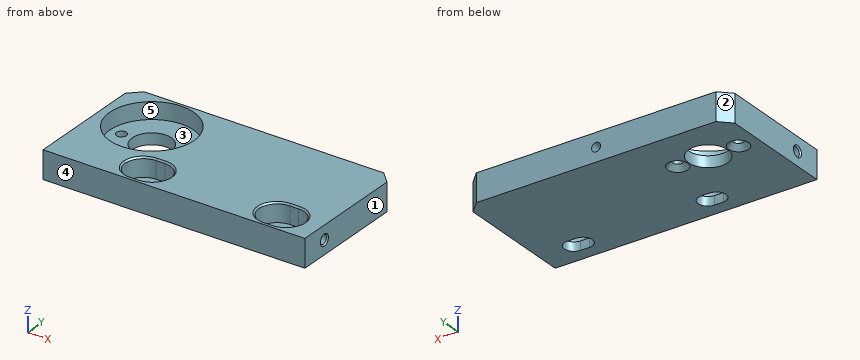
```python
from build123d import *

# Parameters (mm, degrees)
SKIZZE1_W                                            = 47
SKIZZE1_H                                            = 23
AUFSATZ_LINEAR_AUSTRAGEN1_DEPTH                      = 5
SKIZZE2_R                                            = 7.55
SCHNITT_LINEAR_AUSTRAGEN1_DEPTH                      = 3
SKIZZE3_R                                            = 3.5
SCHNITT_LINEAR_AUSTRAGEN2_DEPTH                      = 27.636441204
FORMSENKUNG_F_R_M1_6_SENKSCHRAUBE_MIT_SC_D           = 1.8
FORMSENKUNG_F_R_M1_6_SENKSCHRAUBE_MIT_SC_CSINK_D     = 3.6
FORMSENKUNG_F_R_M1_6_SENKSCHRAUBE_MIT_SC_CSINK_ANGLE = 90
M2_GEWINDEBOHRUNG1_D                                 = 1.6
M2_GEWINDEBOHRUNG1_DEPTH                             = 8
M2_GEWINDEBOHRUNG1_CSINK_D                           = 2.05
M2_GEWINDEBOHRUNG1_CSINK_ANGLE                       = 90
M2_GEWINDEBOHRUNG1_TIP                               = 0.480688495
M2_GEWINDEBOHRUNG2_D                                 = 1.6
M2_GEWINDEBOHRUNG2_DEPTH                             = 8
M2_GEWINDEBOHRUNG2_CSINK_D                           = 2.05
M2_GEWINDEBOHRUNG2_CSINK_ANGLE                       = 90
M2_GEWINDEBOHRUNG2_TIP                               = 0.480688495
M2_GEWINDEBOHRUNG3_D                                 = 1.6
M2_GEWINDEBOHRUNG3_DEPTH                             = 8
M2_GEWINDEBOHRUNG3_TIP                               = 0.480688495
FASE1_SIZE                                           = 2
STIRNSENKUNG_START                                   = 1.6
STIRNSENKUNG_LANGLOCH_F_R_M3_ZYLINDERSCH_DEPTH       = 3.4
STIRNSENKUNG_START_2                                 = -1
STIRNSENKUNG_LANGLOCH_F_R_M3_ZYLINDE_3_DEPTH         = 2.6


with BuildPart() as part:
    # Skizze1 → Aufsatz-Linear austragen1 (new body)
    with BuildSketch(Plane.XY):
        Rectangle(SKIZZE1_W, SKIZZE1_H)
    extrude(amount=AUFSATZ_LINEAR_AUSTRAGEN1_DEPTH)

    # Skizze2 → Schnitt-Linear austragen1 (cut)
    with BuildSketch(Plane.XY.offset(5)):
        with Locations((-14.5, 3.5)):
            Circle(SKIZZE2_R)
    extrude(amount=-SCHNITT_LINEAR_AUSTRAGEN1_DEPTH, mode=Mode.SUBTRACT)

    # Skizze3 → Schnitt-Linear austragen2 (cut, through all)
    with BuildSketch(Plane.XY.offset(5)):
        with Locations((-14.5, 3.5)):
            Circle(SKIZZE3_R)
    extrude(amount=-SCHNITT_LINEAR_AUSTRAGEN2_DEPTH, mode=Mode.SUBTRACT)

    # Formsenkung für M1.6 Senkschraube mit Schlitz/Kreuzschlitz1 (through all)
    with Locations(Plane(origin=(0, 0, 0), x_dir=(-1, 0, 0), z_dir=(0, 0, -1))):
        with Locations((9.04, 3.5), (19.96, 3.5)):
            CounterSinkHole(FORMSENKUNG_F_R_M1_6_SENKSCHRAUBE_MIT_SC_D / 2, FORMSENKUNG_F_R_M1_6_SENKSCHRAUBE_MIT_SC_CSINK_D / 2, counter_sink_angle=FORMSENKUNG_F_R_M1_6_SENKSCHRAUBE_MIT_SC_CSINK_ANGLE)

    # M2 Gewindebohrung1
    with Locations(Plane.ZY.offset(23.5)):
        with Locations((2.5, -6.5)):
            CounterSinkHole(M2_GEWINDEBOHRUNG1_D / 2, M2_GEWINDEBOHRUNG1_CSINK_D / 2, depth=M2_GEWINDEBOHRUNG1_DEPTH, counter_sink_angle=M2_GEWINDEBOHRUNG1_CSINK_ANGLE)
            with Locations((0, 0, -(M2_GEWINDEBOHRUNG1_DEPTH + M2_GEWINDEBOHRUNG1_TIP / 2))):  # 118° drill point
                Cone(0, M2_GEWINDEBOHRUNG1_D / 2, M2_GEWINDEBOHRUNG1_TIP, mode=Mode.SUBTRACT)

    # M2 Gewindebohrung2
    with Locations(Plane(origin=(23.5, 0, 0), x_dir=(0, 0, -1), z_dir=(1, 0, 0))):
        with Locations((-2.5, -6.5)):
            CounterSinkHole(M2_GEWINDEBOHRUNG2_D / 2, M2_GEWINDEBOHRUNG2_CSINK_D / 2, depth=M2_GEWINDEBOHRUNG2_DEPTH, counter_sink_angle=M2_GEWINDEBOHRUNG2_CSINK_ANGLE)
            with Locations((0, 0, -(M2_GEWINDEBOHRUNG2_DEPTH + M2_GEWINDEBOHRUNG2_TIP / 2))):  # 118° drill point
                Cone(0, M2_GEWINDEBOHRUNG2_D / 2, M2_GEWINDEBOHRUNG2_TIP, mode=Mode.SUBTRACT)

    # M2 Gewindebohrung3
    with Locations(Plane(origin=(0, 11.5, 0), x_dir=(1, 0, 0), z_dir=(0, 1, 0))):
        with Locations((0, -2.5)):
            Hole(M2_GEWINDEBOHRUNG3_D / 2, depth=M2_GEWINDEBOHRUNG3_DEPTH)
            with Locations((0, 0, -(M2_GEWINDEBOHRUNG3_DEPTH + M2_GEWINDEBOHRUNG3_TIP / 2))):  # 118° drill point
                Cone(0, M2_GEWINDEBOHRUNG3_D / 2, M2_GEWINDEBOHRUNG3_TIP, mode=Mode.SUBTRACT)

    # Fase1
    fase1_edges = [part.edges().sort_by_distance(p)[0] for p in [
        (-23.5, 11.5, 2.5),
        (23.5, 11.5, 2.5),
    ]]
    chamfer(fase1_edges, length=FASE1_SIZE)

    # Stirnsenkung Langloch für M3 Zylinderschraube mit Innensechskant2: read off the stored shape, not the designer's step
    # Stirnsenkung Langloch f_r M3 Zylinde 2 → Stirnsenkung Langloch für M3 Zylinderschraube mit Innensechskant2 (cut)
    with BuildSketch(Plane.XY.offset(STIRNSENKUNG_START)):
        with BuildLine():
            Line((-8.3, -10.75), (-6.7, -10.75))
            ThreePointArc((-6.7, -10.75), (-3.45, -7.5), (-6.7, -4.25))
            Line((-6.7, -4.25), (-8.3, -4.25))
            ThreePointArc((-8.3, -4.25), (-11.55, -7.5), (-8.3, -10.75))
        make_face()
        with BuildLine():
            ThreePointArc((17.3, -10.75), (20.55, -7.5), (17.3, -4.25))
            Line((17.3, -4.25), (15.7, -4.25))
            ThreePointArc((15.7, -4.25), (12.45, -7.5), (15.7, -10.75))
            Line((15.7, -10.75), (17.3, -10.75))
        make_face()
    extrude(amount=STIRNSENKUNG_LANGLOCH_F_R_M3_ZYLINDERSCH_DEPTH, mode=Mode.SUBTRACT)

    # Stirnsenkung Langloch f_r M3 Zylinde 3 o → Stirnsenkung Langloch f_r M3 Zylinde 3 (cut)
    with BuildSketch(Plane.XY.offset(STIRNSENKUNG_START_2)):
        with BuildLine():
            Line((-8.3, -9.2), (-6.7, -9.2))
            ThreePointArc((-6.7, -9.2), (-5, -7.5), (-6.7, -5.8))
            Line((-6.7, -5.8), (-8.3, -5.8))
            ThreePointArc((-8.3, -5.8), (-10, -7.5), (-8.3, -9.2))
        make_face()
        with BuildLine():
            ThreePointArc((17.3, -9.2), (19, -7.5), (17.3, -5.8))
            Line((17.3, -5.8), (15.7, -5.8))
            ThreePointArc((15.7, -5.8), (14, -7.5), (15.7, -9.2))
            Line((15.7, -9.2), (17.3, -9.2))
        make_face()
    extrude(amount=STIRNSENKUNG_LANGLOCH_F_R_M3_ZYLINDE_3_DEPTH, mode=Mode.SUBTRACT)

    # Stirnsenkung Langloch f_r M3 Zylinde 4: loft between two sections, ruled curve by curve
    stirnsenkung_langloch_f_r_m3_zylinde_4_from = [
        Edge.make_three_point_arc((-6.7, -10.75, 4.725), (-4.401902961, -9.798097039, 4.725), (-3.45, -7.5, 4.725)),
        Edge.make_three_point_arc((-3.45, -7.5, 4.725), (-4.401902961, -5.201902961, 4.725), (-6.7, -4.25, 4.725)),
        Edge.make_three_point_arc((-8.3, -4.25, 4.725), (-10.598097039, -5.201902961, 4.725), (-11.55, -7.5, 4.725)),
        Edge.make_three_point_arc((-11.55, -7.5, 4.725), (-10.598097039, -9.798097039, 4.725), (-8.3, -10.75, 4.725)),
        Edge.make_line((-6.7, -4.25, 4.725), (-8.3, -4.25, 4.725)),
        Edge.make_line((-6.7, -10.75, 4.725), (-8.3, -10.75, 4.725)),
    ]
    stirnsenkung_langloch_f_r_m3_zylinde_4_to = [
        Edge.make_three_point_arc((-6.7, -11.025, 5), (-4.207448596, -9.992551404, 5), (-3.175, -7.5, 5)),
        Edge.make_three_point_arc((-3.175, -7.5, 5), (-4.207448596, -5.007448596, 5), (-6.7, -3.975, 5)),
        Edge.make_three_point_arc((-8.3, -3.975, 5), (-10.792551404, -5.007448596, 5), (-11.825, -7.5, 5)),
        Edge.make_three_point_arc((-11.825, -7.5, 5), (-10.792551404, -9.992551404, 5), (-8.3, -11.025, 5)),
        Edge.make_line((-6.7, -3.975, 5), (-8.3, -3.975, 5)),
        Edge.make_line((-6.7, -11.025, 5), (-8.3, -11.025, 5)),
    ]
    stirnsenkung_langloch_f_r_m3_zylinde_4 = Solid(Shell([*[Face.make_surface_from_curves(stirnsenkung_langloch_f_r_m3_zylinde_4_from[k], stirnsenkung_langloch_f_r_m3_zylinde_4_to[k]) for k in range(6)], Face(Wire(stirnsenkung_langloch_f_r_m3_zylinde_4_from)), Face(Wire(stirnsenkung_langloch_f_r_m3_zylinde_4_to))]))
    add(stirnsenkung_langloch_f_r_m3_zylinde_4, mode=Mode.SUBTRACT)

    # Stirnsenkung Langloch f_r M3 Zylinde 5: loft between two sections, ruled curve by curve
    stirnsenkung_langloch_f_r_m3_zylinde_5_from = [
        Edge.make_three_point_arc((17.3, -10.75, 4.725), (19.598097039, -9.798097039, 4.725), (20.55, -7.5, 4.725)),
        Edge.make_three_point_arc((20.55, -7.5, 4.725), (19.598097039, -5.201902961, 4.725), (17.3, -4.25, 4.725)),
        Edge.make_three_point_arc((15.7, -4.25, 4.725), (13.401902961, -5.201902961, 4.725), (12.45, -7.5, 4.725)),
        Edge.make_three_point_arc((12.45, -7.5, 4.725), (13.401902961, -9.798097039, 4.725), (15.7, -10.75, 4.725)),
        Edge.make_line((17.3, -4.25, 4.725), (15.7, -4.25, 4.725)),
        Edge.make_line((17.3, -10.75, 4.725), (15.7, -10.75, 4.725)),
    ]
    stirnsenkung_langloch_f_r_m3_zylinde_5_to = [
        Edge.make_three_point_arc((17.3, -11.025, 5), (19.792551404, -9.992551404, 5), (20.825, -7.5, 5)),
        Edge.make_three_point_arc((20.825, -7.5, 5), (19.792551404, -5.007448596, 5), (17.3, -3.975, 5)),
        Edge.make_three_point_arc((15.7, -3.975, 5), (13.207448596, -5.007448596, 5), (12.175, -7.5, 5)),
        Edge.make_three_point_arc((12.175, -7.5, 5), (13.207448596, -9.992551404, 5), (15.7, -11.025, 5)),
        Edge.make_line((17.3, -3.975, 5), (15.7, -3.975, 5)),
        Edge.make_line((17.3, -11.025, 5), (15.7, -11.025, 5)),
    ]
    stirnsenkung_langloch_f_r_m3_zylinde_5 = Solid(Shell([*[Face.make_surface_from_curves(stirnsenkung_langloch_f_r_m3_zylinde_5_from[k], stirnsenkung_langloch_f_r_m3_zylinde_5_to[k]) for k in range(6)], Face(Wire(stirnsenkung_langloch_f_r_m3_zylinde_5_from)), Face(Wire(stirnsenkung_langloch_f_r_m3_zylinde_5_to))]))
    add(stirnsenkung_langloch_f_r_m3_zylinde_5, mode=Mode.SUBTRACT)


solid = part.part
```
Can you work these out from the model? Positions are in its coordinate system, mm. Face numbers are marked on the shaded views. A direction names the side the tool comes from. Round coordinates to 2 decimals unless told otherwise and drop trailing zeros. Order: outer loops, then holes, each group sorted by start corner. A loop starts at its lowest first (then second) coordinate and runs counter-clockwise, first axis right, second up. Notation, with made-up numbers: (-26.75, 0) -> (21.25, 0) arc R31 ccw to (21.25, 39) -> close; hole circle Ø3 at (40, -2.75). An arc over 180 degrees is marked (long way). Return JSON: item names as keys, results as strings. Group by question number.
1. If we section it at B-B, the plane x = -19.96: Write out the boundary of the cut face in (y, z), then the cut area to 3 significant figures.
2. If we section it at A-A, the plane x = -14.5: Write out the boundary of the cut face in (y, z), then the cut area to 3 significant figures.
3. I need wall thicknesses on line 1 (X direction, y = 7.5, z = 2.5); line 2 (Z direction, x = 22.6, y = -6.5); line 3 (Y direction, x = 20.8, z = 2.5). Which ranges of each line are inside material? Lowest first, please. Write a range as [from, to].
4. Will these pins go through, and if not, where does the flat tip stop? pin 1 (8 mm diameter, centred on x = -14.5, y = 3.5, fed in from +Z); pin 2 (1.4 mm diameter, centred on y = -6.5, z = 2.5, fed in from -X).
5. Which directions (+Z, -Z, +X, -X, +Y, -Y) give clear straight access to the entire face, cutting with the end or side of a thin tool? Please do the marked faces 4 and 5.
6. We'd pull the mould along Y, two halves only. Please class the marked faces 1, 2 and 3: released by +Y, released by -Y, zero draft, split by the parting line, or undercut.
7. If we section it at C-C, the plane y = 1.25: Write out the boundary of the cut face in (x, z), then the cut area to 3 significant figures.
8. If we section it at D-D, the plane y = 10.25: Write out the boundary of the cut face in (x, z).
Output values:
{
 "1": {"outline": "(-11.5, 0) -> (1.7, 0) -> (2.6, 0.9) -> (2.6, 2) -> (-1.71, 2) -> (-1.71, 5) -> (-11.5, 5) -> close; (4.4, 0.9) -> (5.3, 0) -> (11.5, 0) -> (11.5, 5) -> (8.71, 5) -> (8.71, 2) -> (4.4, 2) -> close; hole circle Ø1.6 at (-6.5, 2.5)", "area": "77.3 mm²"},
 "2": {"outline": "(-11.5, 0) -> (0, 0) -> (0, 2) -> (-4.05, 2) -> (-4.05, 5) -> (-11.5, 5) -> close; (7, 0) -> (11.5, 0) -> (11.5, 5) -> (11.05, 5) -> (11.05, 2) -> (7, 2) -> close", "area": "55.7 mm²"},
 "3": {"line 1": "[-23.5, -20.9], [-8.1, -0.8], [0.8, 23.5]", "line 2": "[0, 1.7], [3.3, 5]", "line 3": "[-11.5, -7.3], [-5.7, 11.5]"},
 "4": {"pin 1": "z = 2", "pin 2": "x = -15.44"},
 "5": {"face 4": "+Z, -Z, +X, -X, -Y", "face 5": "+Z"},
 "6": {"face 1": "zero draft", "face 2": "released by +Y", "face 3": "undercut"},
 "7": {"outline": "(-23.5, 0) -> (-17.18, 0) -> (-17.18, 2) -> (-21.71, 2) -> (-21.71, 5) -> (-23.5, 5) -> close; (-11.82, 0) -> (23.5, 0) -> (23.5, 5) -> (-7.29, 5) -> (-7.29, 2) -> (-11.82, 2) -> close", "area": "181 mm²"},
 "8": {"outline": "(-22.75, 0) -> (22.75, 0) -> (22.75, 5) -> (-11.12, 5) -> (-11.12, 2) -> (-17.88, 2) -> (-17.88, 5) -> (-22.75, 5) -> close; hole circle Ø1.6 at (0, 2.5)"}
}
